Can you work these out from the model? Positions are in its coordinate system, mm. A direction names the side the tool comes from. Give positions to 0.01 mm unless a question says otherwise; leave off trailing zeros. Order: outer loops, then holes, each group sorted by start corner. A loop starts at its lowest first (then second) coordinate and runs counter-clockwise, first axis right, second up. Notation, with made-up numbers: (35.25, -34.5) - (73.25, -34.5) arc R15 ccw to (73.25, -27.5) - close; hole circle Ø2 at (3.25, 39.5). An arc over 180 degrees is marked (long way). Answer as a JSON object with one key per item and string values.
```python
from build123d import *

# Parameters (mm, degrees)
F0_W     = 6
F0_H     = 7
F0_R     = 1.5
F1_DEPTH = 21
F2_W     = 19
F2_H     = 6
F3_DEPTH = 10.4
F4_R     = 1.05
F5_DEPTH = 25


with BuildPart() as f1:
    # F0 (on Front) → F1 (new body)
    with BuildSketch(Plane.XZ):
        with Locations((-3, -3.5)):
            Rectangle(F0_W, F0_H)
        with Locations((-3, -4.5)):
            Circle(F0_R, mode=Mode.SUBTRACT)
    extrude(amount=F1_DEPTH)

    # F2 (on face) → F3 (cut)
    with BuildSketch(Plane.YZ):
        with Locations((-10.5, -4)):
            Rectangle(F2_W, F2_H)
    extrude(amount=-F3_DEPTH, mode=Mode.SUBTRACT)

    # F4 (on face) → F5 (cut)
    with BuildSketch(Plane.XY):
        with Locations((-3, -10.5)):
            Circle(F4_R)
    extrude(amount=-F5_DEPTH, mode=Mode.SUBTRACT)


solid = f1.part
```
Q1. If we section it at D-D, the plane z = -4.5: Please give me the cut outline in (x, y), then the cut area to 3 significant figures.
Recorded:
{"outline": "(-6, -21) - (-4.5, -21) - (-4.5, -20) - (-6, -20) - close; (-6, -1) - (-4.5, -1) - (-4.5, 0) - (-6, 0) - close; (-1.5, -21) - (0, -21) - (0, -20) - (-1.5, -20) - close; (-1.5, -1) - (0, -1) - (0, 0) - (-1.5, 0) - close", "area": "6.00 mm^2"}
Q2. I'm going to push flat-ended pins straight in: pin 1 Ø3 at (x, z) = (-4, -2.5) entering from +Y; pin 2 Ø1 at (x, y) = (-2.5, -17) entering from -Z; pin 3 Ø2.5 at (x, z) = (-3, -4.5) entering from +Y. Where does each tip first touch, or does it pass through?
Recorded:
{"pin 1": "stops at y = 0", "pin 2": "stops at z = -1", "pin 3": "passes through"}
Q3. If we section it at B-B, the plane z = -1.5: Please give me the cut outline in (x, y).
Recorded:
{"outline": "(-6, -21) - (0, -21) - (0, -20) - (-6, -20) - close; (-6, -1) - (0, -1) - (0, 0) - (-6, 0) - close"}
Q4. If we section it at C-C, the plane x = -3: Please give me the cut outline in (y, z), then the cut area to 3 significant figures.
Recorded:
{"outline": "(-21, -7) - (-20, -7) - (-20, -6) - (-21, -6) - close; (-21, -3) - (-20, -3) - (-20, -1) - (-11.55, -1) - (-11.55, 0) - (-21, 0) - close; (-9.45, -1) - (-1, -1) - (-1, -3) - (0, -3) - (0, 0) - (-9.45, 0) - close; (-1, -7) - (0, -7) - (0, -6) - (-1, -6) - close", "area": "24.9 mm^2"}
Q5. I need wall thicknesses on L1, parallel to X at y = -20.7, z = -4.5; L2, parallel to Y at x = -3, z = -0.5; L3, parallel to Y at x = -5.05, z = -3. Which ranges of each line are inside material? Lowest first, please.
Recorded:
{"L1": "x = -6 to -4.5, -1.5 to 0", "L2": "y = -21 to -11.55, -9.45 to 0", "L3": "y = -21 to -20, -1 to 0"}
Q6. Which directions (+Z, -Z, +X, -X, +Y, -Y) give clear straight access to the entire face, cutting with the end or side of a thin tool? Please do faces 1 (the face through (-1.57, -20.49, -4.05)), 2 (the face through (-3, -1, -2.7)).
Recorded:
{"face 1": "+Y, -Y", "face 2": "-Z, +X, -X"}
Q7. If we section it at A-A, the plane y = -10.5: Please give me the cut outline in (x, z).
Recorded:
{"outline": "(-6, -1) - (-4.05, -1) - (-4.05, 0) - (-6, 0) - close; (-1.95, -1) - (0, -1) - (0, 0) - (-1.95, 0) - close"}
Q8. We'd pull the mould along Y, two halves only. Please class faces 3 (the face through (-2.44, -9.61, -0.49)), 4 (the face through (-3, -20.5, -7)), 5 (the face through (-3, -21, -2.7)): released by +Y, released by -Y, zero draft, split by the parting line, or undercut.
Recorded:
{"face 3": "undercut", "face 4": "zero draft", "face 5": "released by -Y"}
